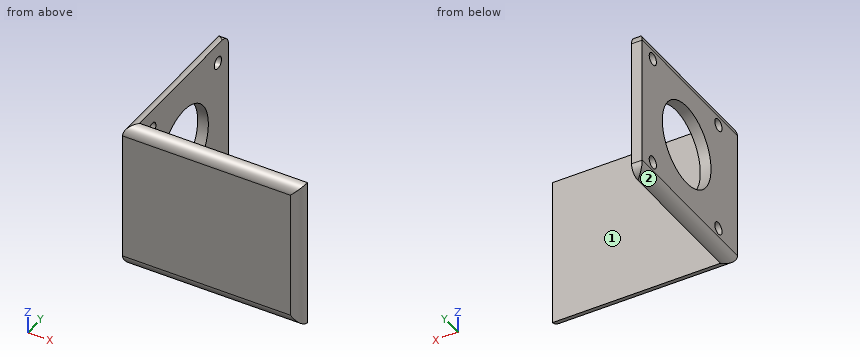
```python
from build123d import *

# Parameters (mm, degrees)
BOSS_EXTRUDE1_DEPTH = 21
FILLET1_R           = 3
SKETCH2_R           = 11.5
SKETCH2_R_2         = 1.7
CUT_EXTRUDE2_DEPTH  = 69.373971656


with BuildPart() as part:
    # Sketch1 → Boss-Extrude1 (new, symmetric)
    with BuildSketch(Plane.XY):
        Polygon((0, 0), (0, 45), (3, 45), (3, 3), (50, 3), (50, 0), align=None)
    extrude(amount=BOSS_EXTRUDE1_DEPTH, both=True)

    # Fillet1
    fillet1_edges = [part.edges().sort_by_distance(p)[0] for p in [
        (0, 22.5, -21),
        (25, 0, -21),
        (50, 0, 0),
        (0, 22.5, 21),
        (25, 0, 21),
        (1.5, 45, -21),
        (1.5, 45, 21),
    ]]
    fillet(fillet1_edges, radius=FILLET1_R - 0.0001)  # a hair under: the kernel refuses the full size

    # Sketch2 → Cut-Extrude2 (cut, through all)
    with BuildSketch(Plane(origin=(3, 0, 0), x_dir=(0, 0, -1), z_dir=(1, 0, 0))):
        with Locations(Location((0, 24, 0), (0, 0, 90))):
            Circle(SKETCH2_R)
        with Locations(Location((-15.5, 40, 0), (0, 0, 90))):
            Circle(SKETCH2_R_2)
        with Locations(Location((-15.5, 9, 0), (0, 0, 270))):
            Circle(SKETCH2_R_2)
        with Locations(Location((15.5, 9, 0), (0, 0, 90))):
            Circle(SKETCH2_R_2)
        with Locations(Location((15.5, 40, 0), (0, 0, 270))):
            Circle(SKETCH2_R_2)
    extrude(amount=-CUT_EXTRUDE2_DEPTH, mode=Mode.SUBTRACT)


solid = part.part
```
Geometry check sheet. Reference: the model listing, model coordinates, mm. Face numbers are marked on the shaded views. A direction names the side the tool comes from. Give positions to 0.01 mm unless a question says otherwise; leave off trailing zeros.
1. Thickness scan on L1, parallel to Y at x = 1, z = 15; L2, parallel to Z at x = 1.55, y = 9; L3, parallel to X at y = 4, z = 16.5. Record the ranges inside material, lowest first.
2. Access from +Z, -Z, +X, -X, +Y, -Y to the whole of each face (thin tool, end or side, straight path). Record for the marked faces 1 and 2.
3. Section check A-A, the plane y = 40. Give the number of separate pieces and of enclosed holes in the cut face, and give its area (3 significant figures).
4. Gauge pin test, flat ends, axial feed: pin 1 Ø5 at (y, z) = (21.5, 9) entering from +X; pin 2 Ø3 at (y, z) = (9, -15.5) entering from +X; pin 3 Ø12.5 at (x, z) = (28.5, 4) entering from +Y. Record the tip position at first contact, or that the pin passes through.
Values follow:
1. L1: y = 0 to 7.38, 10.62 to 38.38, 41.62 to 45
1. L2: z = -20.63 to -17.2, -13.8 to 13.8, 17.2 to 20.63
1. L3: x = 0 to 3
2. face 1: +Z, -Z, +X, +Y
2. face 2: -Z, -X, +Y, -Y
3. separate pieces: 3
3. enclosed holes: 0
3. area: 102 mm2
4. pin 1: stops at x = 3
4. pin 2: passes through
4. pin 3: stops at y = 3
